```python
from build123d import *

# Parameters (mm, degrees)
SALIENTE_EXTRUIR1_DEPTH = 20
CROQUIS2_W              = 3
CROQUIS2_H              = 20
SALIENTE_EXTRUIR2_DEPTH = 3
CROQUIS3_W              = 20
CROQUIS3_H              = 3
SALIENTE_EXTRUIR3_DEPTH = 60
SALIENTE_EXTRUIR4_DEPTH = 9.5
CROQUIS5_W              = 9.5
CROQUIS5_H              = 3.5
SALIENTE_EXTRUIR6_DEPTH = 20
CROQUIS6_R              = 4
CORTAR_EXTRUIR1_DEPTH   = 1.2
CROQUIS7_R              = 1
CORTAR_EXTRUIR2_DEPTH   = 1.8
CROQUIS8_R              = 1
CORTAR_EXTRUIR4_DEPTH   = 6.75


with BuildPart() as part:
    # Croquis1 → Saliente-Extruir1 (new body)
    with BuildSketch(Plane(origin=(0, 0, 0), x_dir=(1, 0, 0), z_dir=(0, 1, 0))):
        Polygon((-63.528635851, -28.815731451), (-2.528635851, -28.815731451), (-2.528635851, 10.784268549), (-5.528635851, 10.784268549), (-5.528635851, -25.815731451), (-63.528635851, -25.815731451), align=None)
    extrude(amount=SALIENTE_EXTRUIR1_DEPTH)

    # Croquis2 → Saliente-Extruir2 (add)
    with BuildSketch(Plane(origin=(0, 20, 0), x_dir=(1, 0, 0), z_dir=(0, 1, 0))):
        with Locations((-4.028635851, 0.784268549)):
            Rectangle(CROQUIS2_W, CROQUIS2_H)
    extrude(amount=SALIENTE_EXTRUIR2_DEPTH)

    # Croquis3 → Saliente-Extruir3 (add)
    with BuildSketch(Plane(origin=(-2.528635851, 0, 0), x_dir=(0, 0, -1), z_dir=(1, 0, 0))):
        with Locations((0.784268549, 21.5)):
            Rectangle(CROQUIS3_W, CROQUIS3_H)
    extrude(amount=SALIENTE_EXTRUIR3_DEPTH)

    # Croquis4 → Saliente-Extruir4 (add)
    with BuildSketch(Plane(origin=(-2.528635851, 0, 0), x_dir=(0, 0, -1), z_dir=(1, 0, 0))):
        Polygon((-9.215731451, 20), (-9.015731451, 0), (-5.515731451, 0), (-5.715731451, 20), align=None)
    extrude(amount=SALIENTE_EXTRUIR4_DEPTH)

    # Croquis5 → Saliente-Extruir6 (add)
    with BuildSketch(Plane.XZ.offset(-20)):
        with Locations((52.721364149, 7.465731451)):
            Rectangle(CROQUIS5_W, CROQUIS5_H)
    extrude(amount=SALIENTE_EXTRUIR6_DEPTH)

    # Croquis6 → Cortar-Extruir1 (cut)
    with BuildSketch(Plane(origin=(0, 0, 25.815731451), x_dir=(-1, 0, 0), z_dir=(0, 0, -1))):
        with Locations((44.528635851, 10)):
            Circle(CROQUIS6_R)
    extrude(amount=-CORTAR_EXTRUIR1_DEPTH, mode=Mode.SUBTRACT)

    # Croquis7 → Cortar-Extruir2 (cut)
    with BuildSketch(Plane(origin=(0, 0, 27.015731451), x_dir=(-1, 0, 0), z_dir=(0, 0, -1))):
        with Locations((44.528635851, 10)):
            Circle(CROQUIS7_R)
    extrude(amount=-CORTAR_EXTRUIR2_DEPTH, mode=Mode.SUBTRACT)

    # Croquis8 → Cortar-Extruir4 (cut, symmetric)
    with BuildSketch(Plane(origin=(0, -0.0901483, 9.014829968), x_dir=(1, 0, 0), z_dir=(0, -0.009999500037496644, 0.9999500037496877))):
        with Locations(Location((2.721364149, 15.340652794, 0), (0, 0, 270))):
            Circle(CROQUIS8_R)
        with Locations(Location((2.721364149, 4.840152807, 0), (0, 0, 270))):
            Circle(CROQUIS8_R)
        with Locations(Location((52.221364149, 15.340652794, 0), (0, 0, 270))):
            Circle(CROQUIS8_R)
        with Locations(Location((52.221364149, 4.840152807, 0), (0, 0, 270))):
            Circle(CROQUIS8_R)
    extrude(amount=CORTAR_EXTRUIR4_DEPTH, both=True, mode=Mode.SUBTRACT)


solid = part.part
```
CAD build for the part. Positions are in the model's coordinates, mm. A direction names the side the tool comes from. Round coordinates to 2 decimals unless told otherwise and drop trailing zeros. Order: outer loops, then holes, each group sorted by start corner. A loop starts at its lowest first (then second) coordinate and runs counter-clockwise, first axis right, second up. Notation, with made-up numbers: (-9, 16.5) - (21, 16.5) arc R24 ccw to (21, 29.5) - close; hole circle Ø4 at (27.25, -30.5). An arc over 180 degrees is marked (long way). Use CSV: the item, a comma, the result in double quotes. Start each with the question number.
1) Saw through at C-C (z = 1). List the corners of the cut face in (x, y), and give its area (3 significant figures).
2) Tool access for faces 1 (the flat face through (57.471, 17, 6)), 2 (the flat face through (47.971, 10, 7)), 3 (the flat face through (53, 10, 5.716)), 4 (the cylindrical face through (-48.344, 11.201, 26.407)), 5 (the flat face through (-5.529, 11, 8)): list every direction of +Z, -Z, +X, -X, +Y, -Y with a clear straight run to the whole face (end or side of a thin tool).
3) Wall check: L1, parallel to X at y = 17, z = 7.5; L2, parallel to X at y = 5.5, z = 7.5; L3, parallel to Z at x = -55.5, y = 11.5. Give the ranges that are in metal, low to high. Write a range as [from, to].
4) Saw through at B-B (z = 13.5). List the corners of the cut face in (x, y).
5) Two-plate mould, pull along X, no slides. Class faces 6 (the flat face through (19, 21, -10.784)), 7 (the flat face through (-2.529, 10, -2)), 8 (the cylindrical face through (51.245, 4.982, 7.493)), 9 (the cylindrical face through (1.83, 4.31, 7.33)): pulls with the +X half, pulls with the -X half, needs draft (parallel to the pull), parting line crosses it, or undercut.
6) Pin check, flat tips, straight feed: pin 1 Ø8 at (y, z) = (6, -6) entering from +X; pin 2 Ø2.5 at (x, y) = (-44.53, 10) entering from -Z; pin 3 Ø11.5 at (y, z) = (11.5, 14.5) entering from -X. Stop position of each tip, or through.
7) Saw through at A-A (x = -51). List the corners of the cut face in (y, z).
Values follow:
1,outline,"(-5.53, 0) - (-2.53, 0) - (-2.53, 20) - (57.47, 20) - (57.47, 23) - (-5.53, 23) - close"
1,area,"249 mm2"
2,face 1,"+Z, -Z, +X, +Y, -Y"
2,face 2,"+Z, -Z, -Y"
2,face 3,"-Z, +X, -Y"
2,face 4,"-Z"
2,face 5,"-Z, -X, +Y, -Y"
3,L1,"x = [-5.53, 6.97], [47.97, 57.47]"
3,L2,"x = [-5.53, 2.04], [3.4, 6.97], [47.97, 51.54], [52.9, 57.47]"
3,L3,"z = [25.82, 28.82]"
4,outline,"(-5.53, 0) - (-2.53, 0) - (-2.53, 20) - (-5.53, 20) - close"
5,face 6,"needs draft"
5,face 7,"pulls with the +X half"
5,face 8,"undercut"
5,face 9,"undercut"
6,pin 1,"stops at x = -2.53"
6,pin 2,"stops at z = 27.02"
6,pin 3,"stops at x = -5.53"
7,outline,"(0, 25.82) - (20, 25.82) - (20, 28.82) - (0, 28.82) - close"
